Geometry: final body of the model. Coordinates: model frame, mm. A direction names the side the tool comes from. Round coordinates to 2 decimals unless told otherwise and drop trailing zeros. Loops run counter-clockwise (first coordinate to the right, second up) from the corner with the lowest first, then second, coordinate; pieces in that order, holes last. Notation, with made-up numbers: (31, -35.75) -> (90, -35.75) arc R18 cw to (90, -28.75) -> close; hole circle Ø11 at (27, 49.25). An arc over 180 degrees is marked (long way). Answer in a Markdown table with one row per item.
```python
from build123d import *

# Parameters (mm, degrees)
F0_W           = 22.3758686334
F0_H           = 16.4037477225
F1_DEPTH       = 254
F2_R           = 5.08
F3_T           = -2.54
F5_DEPTH       = 25.4
F7_D           = 5.5
F7_CSINK_D     = 11.2
F7_CSINK_ANGLE = 90


# Not quite as in the source:
# - a shell that OpenCascade refuses in one call is made with other operations: the cavity is built on its own and cut out


with BuildPart() as f1:
    # F0 (on Front) → F1 (new body)
    with BuildSketch(Plane.XZ):
        with Locations((-11.1879343167, -8.2018738613)):
            Rectangle(F0_W, F0_H)
    extrude(amount=F1_DEPTH)

    # F2
    f2_edges = [f1.edges().sort_by_distance(p)[0] for p in [
        (0, -127, 0),
        (-22.375869, -127, 0),
        (-11.187934, 0, 0),
        (-11.187934, -254, 0),
        (-22.375869, -127, -16.403748),
        (0, -127, -16.403748),
        (-11.187934, 0, -16.403748),
        (-11.187934, -254, -16.403748),
    ]]
    fillet(f2_edges, radius=F2_R)

    # F3: a shell. OpenCascade refuses it in one call, so the cavity is built on its own and cut out:
    # the body offset inwards by the wall thickness, plus a prism from it out through each open face.
    f3_core = offset(f1.part, amount=F3_T, mode=Mode.PRIVATE)
    f3_exits = [f3_core.faces().sort_by_distance(p)[0] for p in [
        (-11.187934, -127, -2.54),
    ]]
    add(f3_core, mode=Mode.SUBTRACT)
    extrude(f3_exits, amount=-F3_T, mode=Mode.SUBTRACT)

    # F4 (on face) → F5 (join)
    with BuildSketch(Plane(origin=(0, 0, -16.4037477225), x_dir=(1, 0, 0), z_dir=(0, 0, -1))):
        Polygon((-14.9793126683, 145.9724638483), (-12.4393126683, 145.9724638483), (-9.8993126683, 145.9724638483), (-12.4393126683, 151.0524716356), align=None)
    extrude(amount=F5_DEPTH)

    # F7 (through all)
    with Locations(Plane(origin=(0, 0, -16.4037477225), x_dir=(1, 0, 0), z_dir=(0, 0, -1))):
        with Locations((-10.6817428023, 79.9587219954)):
            CounterSinkHole(F7_D / 2, F7_CSINK_D / 2, counter_sink_angle=F7_CSINK_ANGLE)


solid = f1.part
```
Item 1: Cut plane A-A (y = -209). Output: boundary loops of the cut face in (x, z), then the cut area to 3 significant figures.
Answer:
| item | result |
|---|---|
| outline | (-22.38, -11.32) arc R5.08 ccw to (-17.3, -16.4) -> (-5.08, -16.4) arc R5.08 ccw to (0, -11.32) -> (0, -5.08) arc R5.08 ccw to (-5.08, 0) -> (-5.08, -2.54) arc R2.54 cw to (-2.54, -5.08) -> (-2.54, -11.32) arc R2.54 cw to (-5.08, -13.86) -> (-17.3, -13.86) arc R2.54 cw to (-19.84, -11.32) -> (-19.84, -5.08) arc R2.54 cw to (-17.3, -2.54) -> (-17.3, 0) arc R5.08 ccw to (-22.38, -5.08) -> close |
| area | 124 mm² |
Item 2: Draft query along X for faces 5 (the face through (-11.03, -252.47, -14.96)), 6 (the face through (-1.449, -128.778, -1.528)), 7 (the face through (-22.376, -125, -8)), 8 (the face through (-19.836, -125, -8)). Return one class per face: pulls with the +X half, pulls with the -X half, needs draft (parallel to the pull), parting line crosses it, or undercut.
Answer:
| item | result |
|---|---|
| face 5 | needs draft |
| face 6 | pulls with the +X half |
| face 7 | pulls with the -X half |
| face 8 | undercut |
Item 3: Reachability of faces 1 (the face through (-11.152, -148.477, -28.926)), 2 (the face through (-13.69, -148.55, -28.93)), 3 (the face through (-2.54, -125, -8)), 4 (the face through (-11.031, -1.528, -1.449)) from +Z, -Z, +X, -X, +Y, -Y: full face, straight path, thin tool, end or side. Return the list, or none.
Answer:
| item | result |
|---|---|
| face 1 | -Z, +X, -Y |
| face 2 | -Z, -X, -Y |
| face 3 | none |
| face 4 | +Z, +X, -X, +Y |
Item 4: Line query: probe 1 along Y at (x, z) = (-7.25, -7); probe 2 along X at (y, z) = (-161, -7.5); probe 3 along Z at (x, y) = (-14.5, -185). Output: solid intervals per line, ascending. Write a range as [from, to].
Answer:
| item | result |
|---|---|
| probe 1 | y = [-254, -251.46], [-2.54, 0] |
| probe 2 | x = [-22.38, -19.84], [-2.54, 0] |
| probe 3 | z = [-16.4, -13.86] |
Item 5: Cut plane B-B (z = -30). Output: boundary loops of the cut face in (x, y).
Answer:
| item | result |
|---|---|
| outline | (-14.98, -145.97) -> (-12.44, -151.05) -> (-9.9, -145.97) -> close |
Item 6: Pin query (flat end, axial travel): pin 1 Ø2 at (x, z) = (-14, -28.5) entering from -Y; pin 2 Ø3 at (x, y) = (-8, -102.5) entering from +Z; pin 3 Ø12 at (y, z) = (-177, -27.5) entering from +X; pin 4 Ø4 at (x, z) = (-13, -23) entering from +Y. Return the tip coordinate at first contact, or that it passes through.
Answer:
| item | result |
|---|---|
| pin 1 | stops at y = -149.93 |
| pin 2 | stops at z = -13.86 |
| pin 3 | passes through |
| pin 4 | stops at y = -145.97 |
